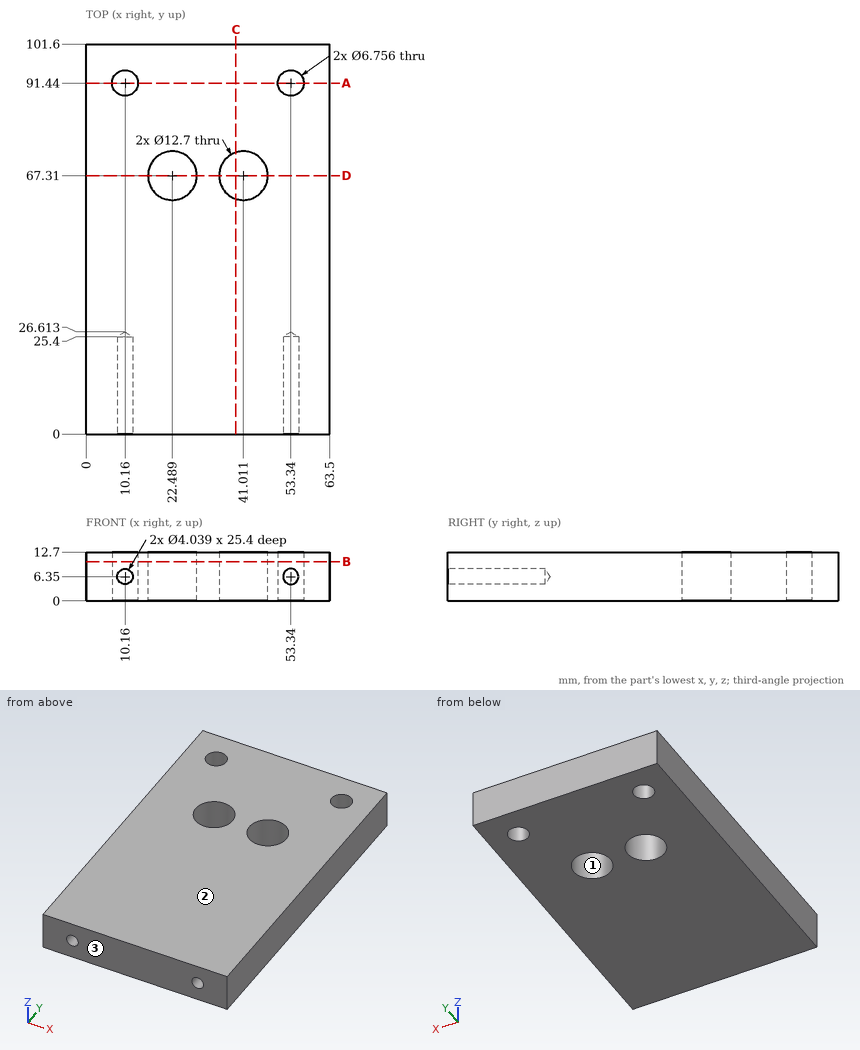
Could you check a few things on this drawing? It's one solid part, dimensions in mm from its lowest x, y, z. Round coordinates to 2 decimals unless told otherwise and drop trailing zeros. Order: outer loops, then holes, each group sorted by start corner. A loop starts at its lowest first (then second) coordinate and runs counter-clockwise, first axis right, second up. Notation, with made-up numbers: M -21.5,-8 L 14.5,-8 A22 ccw 14.5,14 Z; hole C 74,-38.75 d7. An arc over 180 degrees is marked long. Use a Markdown table: item, result.
1) I'm going to push a flat-ended pin straight in: P1, Ø3, axis at x = 53.34, z = 6.35, coming from the -Y side. Where does the tip first touch, or does it pass through?
Geometry says:
| item | result |
|---|---|
| P1 | stops at y = 25.71 |
2) Imagine slicing it at C-C (x = 39). List the corners of the cut face in (y, z) for me.
Geometry says:
| item | result |
|---|---|
| outline | M 0,0 L 61.29,0 L 61.29,12.7 L 0,12.7 Z; M 73.33,0 L 101.6,0 L 101.6,12.7 L 73.33,12.7 Z |
3) Imagine slicing it at A-A (y = 91.44). List the corners of the cut face in (x, z) for me, then the cut area to 3 significant figures.
Geometry says:
| item | result |
|---|---|
| outline | M 0,0 L 6.78,0 L 6.78,12.7 L 0,12.7 Z; M 13.54,0 L 49.96,0 L 49.96,12.7 L 13.54,12.7 Z; M 56.72,0 L 63.5,0 L 63.5,12.7 L 56.72,12.7 Z |
| area | 635 mm² |
4) Imagine slicing it at B-B (z = 10.25). List the corners of the cut face in (x, y) for me.
Geometry says:
| item | result |
|---|---|
| outline | M 0,0 L 63.5,0 L 63.5,101.6 L 0,101.6 Z; hole C 10.16,91.44 d6.76; hole C 22.49,67.31 d12.7; hole C 41.01,67.31 d12.7; hole C 53.34,91.44 d6.76 |
5) If I drill on line 1 along X through (y, z) = (14.25, 6.35); line 2 along Y through (x, z) = (53.5, 2.25) (1 decimal); line 3 along Z through (x, y) = (10.16, 17), over which ranges is the centre line in solid material (lowest first)?
Geometry says:
| item | result |
|---|---|
| line 1 | x = 0 to 8.14, 12.18 to 51.32, 55.36 to 63.5 |
| line 2 | y = 0 to 88.1, 94.8 to 101.6 |
| line 3 | z = 0 to 4.33, 8.37 to 12.7 |
6) Imagine slicing it at D-D (y = 67.31). List the corners of the cut face in (x, z) for me, then the cut area to 3 significant figures.
Geometry says:
| item | result |
|---|---|
| outline | M 0,0 L 16.14,0 L 16.14,12.7 L 0,12.7 Z; M 28.84,0 L 34.66,0 L 34.66,12.7 L 28.84,12.7 Z; M 47.36,0 L 63.5,0 L 63.5,12.7 L 47.36,12.7 Z |
| area | 484 mm² |
7) If we mould it in two halves opening along Y, with no side actions, what happens to the marked faces 1, 2 and 3? For each: +Y half, -Y half, draft (parallel to the pull), parting line (faces both ways), or undercut.
Geometry says:
| item | result |
|---|---|
| face 1 | undercut |
| face 2 | draft |
| face 3 | -Y half |
